```python
from build123d import *

# Parameters (mm, degrees)
SKETCH1_W                              = 50
SKETCH1_H                              = 50
BOSS_EXTRUDE1_DEPTH                    = 8
CBORE_FOR_M6_HEX_HEAD_BOLT2_AT_2_COUNT = 2
CBORE_FOR_M6_HEX_HEAD_BOLT2_AT_2_PITCH = 24


with BuildPart() as part:
    # Sketch1 → Boss-Extrude1 (new body)
    with BuildSketch(Plane.XY):
        Rectangle(SKETCH1_W, SKETCH1_H)
    extrude(amount=BOSS_EXTRUDE1_DEPTH)

    # Sketch14 → CBORE for M6 Hex Head Bolt2 (revolve, cut)
    with BuildSketch(Plane(origin=(0, -12, 8), x_dir=(0, -1, 0), z_dir=(1, 0, 0))):
        Polygon((0, 0), (0, 8), (3.15, 8), (3.15, 4), (6, 4), (6, 1.2985), (7.2985, 0), align=None)
    cbore_for_m6_hex_head_bolt2 = revolve(axis=Axis((0, -12, 14.35), (0, 0, -1)), mode=Mode.SUBTRACT)

    # CBORE for M6 Hex Head Bolt2 at 2: CBORE for M6 Hex Head Bolt2 ×2
    with Locations(*[(0, i * CBORE_FOR_M6_HEX_HEAD_BOLT2_AT_2_PITCH, 0) for i in range(1, CBORE_FOR_M6_HEX_HEAD_BOLT2_AT_2_COUNT)]):
        add(cbore_for_m6_hex_head_bolt2, mode=Mode.SUBTRACT)


solid = part.part
```
For this review, take the finished solid that the model builds, in its own axes (mm). A direction names the side the tool comes from. Give positions to 0.01 mm unless a question says otherwise; leave off trailing zeros. Write each loop counter-clockwise with the first axis right and the second up, starting at its lowest first coordinate (ties: lowest second). Pieces come first, ordered by that corner, then holes.
Item 1: The part is to be moulded in two halves that separate along X. For faces 3 (the face through (25, 0, 4)), 4 (the face through (-0.138, -8.853, 2.028)), 5 (the face through (-25, 0, 4)), 6 (the face through (0, 0, 0)), say which applies: +X half, -X half, draft (parallel to the pull), parting line (faces both ways), or undercut.
Item 2: Take a section at C-C (z = 1.5). Give the boundary of the cut face in (x, y).
Item 3: Insertion check: P1, Ø13, axis at x = -2, y = 10.5, coming from the +Z side; P2, Ø10, axis at x = 0, y = 12, coming from the +Z side. Each pin has a flat end and moves straight along its axis. Give the tip position at first contact, or say it passes through.
Item 4: Take a section at B-B (y = 12). Give the boundary of the cut face in (x, z).
Item 5: Machinability: for faces 1 (the face through (-0.138, 15.147, 2.028)), 2 (the face through (3, -9, 4)), which of the approach directions +Z, -Z, +X, -X, +Y, -Y give a long, thin tool a straight path to every point of the face, cutting with its end or side? Answer none if there is none.
Item 6: Wall thickness on probe 1 along Y at (x, z) = (0, 1.1); probe 2 along X at (y, z) = (12, 5.75); probe 3 along Y at (x, z) = (2, 5): over which ranges is each line inside the solid? List them lowest first.
Item 7: Take a section at A-A (x = 0). Give the boundary of the cut face in (y, z).
Established:
1. face 3: +X half
1. face 4: undercut
1. face 5: -X half
1. face 6: draft
2. outline: (-25, -25) - (25, -25) - (25, 25) - (-25, 25) - close; hole circle Ø6.3 at (0, -12); hole circle Ø6.3 at (0, 12)
3. P1: stops at z = 8
3. P2: stops at z = 4
4. outline: (-25, 0) - (-3.15, 0) - (-3.15, 4) - (-6, 4) - (-6, 6.7) - (-7.3, 8) - (-25, 8) - close; (3.15, 0) - (25, 0) - (25, 8) - (7.3, 8) - (6, 6.7) - (6, 4) - (3.15, 4) - close
5. face 1: +Z, -Z
5. face 2: +Z
6. probe 1: y = -25 to -15.15, -8.85 to 8.85, 15.15 to 25
6. probe 2: x = -25 to -6, 6 to 25
6. probe 3: y = -25 to -17.66, -6.34 to 6.34, 17.66 to 25
7. outline: (-25, 0) - (-15.15, 0) - (-15.15, 4) - (-18, 4) - (-18, 6.7) - (-19.3, 8) - (-25, 8) - close; (-8.85, 0) - (8.85, 0) - (8.85, 4) - (6, 4) - (6, 6.7) - (4.7, 8) - (-4.7, 8) - (-6, 6.7) - (-6, 4) - (-8.85, 4) - close; (15.15, 0) - (25, 0) - (25, 8) - (19.3, 8) - (18, 6.7) - (18, 4) - (15.15, 4) - close
